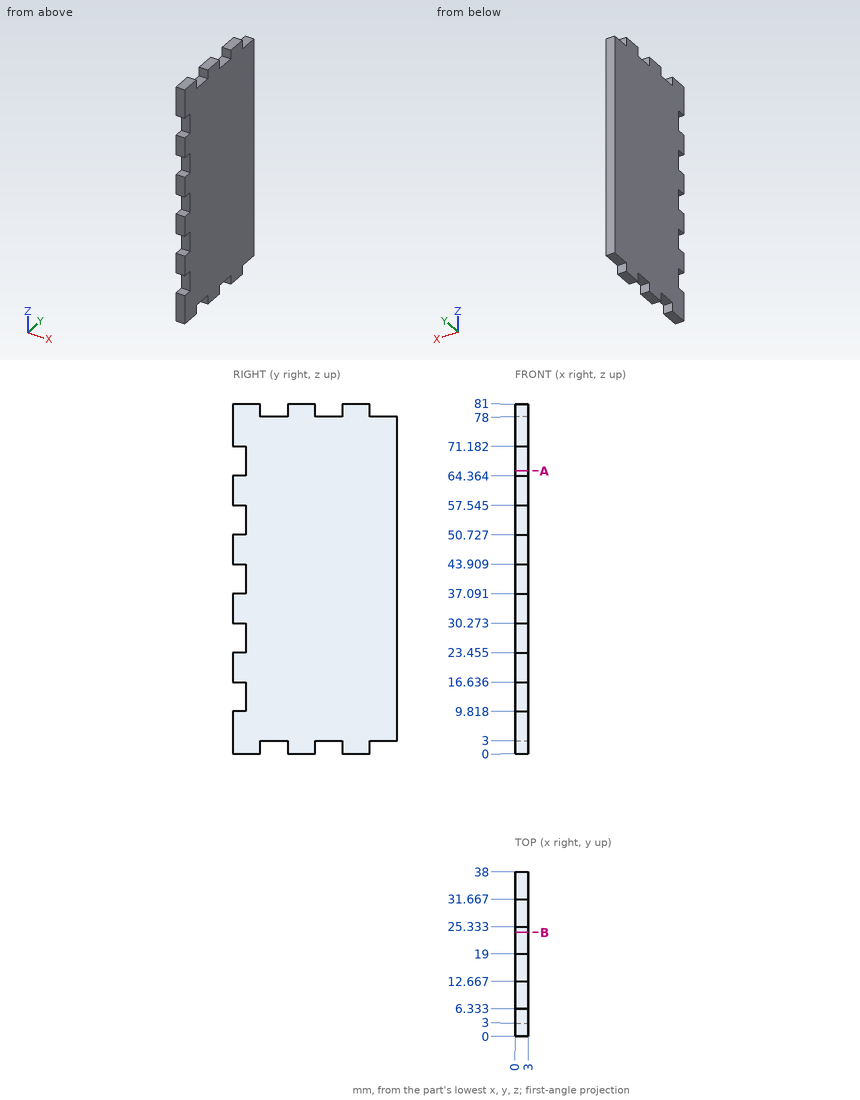
The drawing under review shows one solid part. Ordinate dimensions are in mm from its lowest x, y, z. Round coordinates to 2 decimals unless told otherwise and drop trailing zeros. Order: outer loops, then holes, each group sorted by start corner. A loop starts at its lowest first (then second) coordinate and runs counter-clockwise, first axis right, second up. Notation, with made-up numbers: (-32.5, 54) -> (-9.5, 54) arc R23 cw to (-9.5, 86) -> close; hole circle Ø8 at (2, 53). An arc over 180 degrees is marked (long way). Use a Markdown table: item, result.
Item 1: For line 1 along Z through (x, y) = (0.65, 11.5); line 2 along Y through (x, z) = (2.65, 27), list the stretches that pass through material, from the lowest coordinate up. Write a range as [from, to].
Resolved:
| item | result |
|---|---|
| line 1 | z = [3, 78] |
| line 2 | y = [3, 38] |
Item 2: Take a section at B-B (y = 24). State the section outline as (x, z) points, plus the area to 3 significant figures.
Resolved:
| item | result |
|---|---|
| outline | (0, 3) -> (3, 3) -> (3, 78) -> (0, 78) -> close |
| area | 225 mm² |
Item 3: For pin 1 (3 mm diameter, centred on y = 12.5, z = 49.5, fed in from -X); pin 2 (1.5 mm diameter, centred on x = 2, z = 14.5, fed in from -Y); pin 3 (0.9 mm diameter, centred on x = 1, y = 35, fed in from -Z), all flat-tipped, find the tip position at first contact; note any pin that passes through.
Resolved:
| item | result |
|---|---|
| pin 1 | stops at x = 0 |
| pin 2 | stops at y = 3 |
| pin 3 | stops at z = 3 |
Item 4: Take a section at A-A (z = 65.5). State the section outline as (x, y) points.
Resolved:
| item | result |
|---|---|
| outline | (0, 3) -> (3, 3) -> (3, 38) -> (0, 38) -> close |
